Here's how the part is built. I have some questions about the finished solid (model axes, mm). A direction names the side the tool comes from. Coordinates: 2 decimals unless noted, no trailing zeros. Write each loop counter-clockwise with the first axis right and the second up, starting at its lowest first coordinate (ties: lowest second). Pieces come first, ordered by that corner, then holes. Notation, with made-up numbers: (22.25, 64) -> (57.25, 64) arc R11 ccw to (57.25, 71) -> close; hole circle Ø8 at (84.5, -25). An arc over 180 degrees is marked (long way). Use a Markdown table: item, result. Add a question column.
Item 1: If I drill on line 1 along X through (y, z) = (-23.5, -3.75); line 2 along Y through (x, z) = (0, -1.65); line 3 along X through (y, z) = (16, -1), over which ranges is the centre line in solid material (lowest first)? Write a range as from..to.
Item 2: Imagine slicing it at D-D, the plane y = 16. Write out the boundary of the cut face in (x, z).
Item 3: Will these pins go through, and if not, where does the flat tip stop? pin 1 Ø3 at (x, z) = (-37.5, -5) entering from -Y; pin 2 Ø4 at (x, z) = (36.5, -2) entering from +Y.
Item 4: On a 3-axis mill with a long thin cutter (end or side, diameter ignored), from which of +Z, -Z, +X, -X, +Y, -Y can I reach the whole of each face in a straight line? I mean faces 1 (the flat face through (13, -40, -4)), 2 (the cylindrical face through (-27.496, -24.628, -3.944)). Say none if no direction works.
Item 5: If we mould it in two halves opening along X, with no side actions, what happens to faces 3 (the cylindrical face through (20.21, -9.15, -3.94)), 4 (the flat face through (-1, -46, 0)), 5 (the cylindrical face through (-55.55, -42.594, -3.944))? For each: pulls with the +X half, pulls with the -X half, needs draft (parallel to the pull), parting line crosses it, or undercut.
Item 6: Imagine slicing it at A-A, the plane z = -2. Count the separate pieces of the cut face and the enclosed holes in it, and give its area (3 significant figures).
Item 7: Imagine slicing it at C-C, the plane x = 32. Write out the boundary of the cut face in (y, z), and give its area (3 significant figures).
Item 8: Imagine slicing it at B-B, the plane y = 0. Write out the boundary of the cut face in (x, z), and give its area (3 significant figures).
```python
from build123d import *

# Parameters (mm, degrees)
SKETCH_1_R          = 70
SKETCH_1_R_2        = 17.7
SKETCH_1_R_3        = 2.75
SKETCH_1_R_4        = 1.5
EXTRUDE_1_DEPTH     = 8
SKETCH_2_R          = 45.2
SKETCH_2_R_2        = 41.8
CUT_EXTRUDE_2_DEPTH = 4


with BuildPart() as part:
    # 草图1 → 凸台-拉伸1 (new body)
    with BuildSketch(Plane.XY):
        Circle(SKETCH_1_R)
        Circle(SKETCH_1_R_2, mode=Mode.SUBTRACT)
        with Locations((24.748737342, 24.748737342)):
            Circle(SKETCH_1_R_3, mode=Mode.SUBTRACT)
        with Locations((-24.748737342, 24.748737342)):
            Circle(SKETCH_1_R_3, mode=Mode.SUBTRACT)
        with Locations((-24.748737342, -24.748737342)):
            Circle(SKETCH_1_R_3, mode=Mode.SUBTRACT)
        with Locations((24.748737342, -24.748737342)):
            Circle(SKETCH_1_R_3, mode=Mode.SUBTRACT)
        with Locations((0, 23.75)):
            Circle(SKETCH_1_R_3, mode=Mode.SUBTRACT)
        with Locations((-20.56810334, -11.875)):
            Circle(SKETCH_1_R_3, mode=Mode.SUBTRACT)
        with Locations((20.56810334, -11.875)):
            Circle(SKETCH_1_R_3, mode=Mode.SUBTRACT)
        with Locations((0, 48)):
            Circle(SKETCH_1_R_4, mode=Mode.SUBTRACT)
    extrude(amount=-EXTRUDE_1_DEPTH)

    # 草图2 → 切除-拉伸2 (cut)
    with BuildSketch(Plane.XY):
        Circle(SKETCH_2_R)
        Circle(SKETCH_2_R_2, mode=Mode.SUBTRACT)
    extrude(amount=-CUT_EXTRUDE_2_DEPTH, mode=Mode.SUBTRACT)


solid = part.part
```
Ans:
| question | item | result |
|---|---|---|
| 1 | line 1 | x = -65.94..-38.61, -34.57..-27.2, -22.3..22.3, 27.2..34.57, 38.61..65.94 |
| 1 | line 2 | y = -70..-45.2, -41.8..-17.7, 17.7..21, 26.5..41.8, 45.2..46.5, 49.5..70 |
| 1 | line 3 | x = -68.15..-42.27, -38.62..-7.57, 7.57..38.62, 42.27..68.15 |
| 2 | outline | (-68.15, -8) -> (-7.57, -8) -> (-7.57, 0) -> (-38.62, 0) -> (-38.62, -4) -> (-42.27, -4) -> (-42.27, 0) -> (-68.15, 0) -> close; (7.57, -8) -> (68.15, -8) -> (68.15, 0) -> (42.27, 0) -> (42.27, -4) -> (38.62, -4) -> (38.62, 0) -> (7.57, 0) -> close |
| 3 | pin 1 | stops at y = -60.03 |
| 3 | pin 2 | stops at y = 60.91 |
| 4 | face 1 | +Z |
| 4 | face 2 | +Z, -Z |
| 5 | face 3 | undercut |
| 5 | face 4 | needs draft |
| 5 | face 5 | parting line crosses it |
| 6 | separate pieces | 2 |
| 6 | enclosed holes | 10 |
| 6 | area | 13,300 mm^2 |
| 7 | outline | (-62.26, -8) -> (62.26, -8) -> (62.26, 0) -> (31.92, 0) -> (31.92, -4) -> (26.89, -4) -> (26.89, 0) -> (-26.89, 0) -> (-26.89, -4) -> (-31.92, -4) -> (-31.92, 0) -> (-62.26, 0) -> close |
| 7 | area | 956 mm^2 |
| 8 | outline | (-70, -8) -> (-17.7, -8) -> (-17.7, 0) -> (-41.8, 0) -> (-41.8, -4) -> (-45.2, -4) -> (-45.2, 0) -> (-70, 0) -> close; (17.7, -8) -> (70, -8) -> (70, 0) -> (45.2, 0) -> (45.2, -4) -> (41.8, -4) -> (41.8, 0) -> (17.7, 0) -> close |
| 8 | area | 810 mm^2 |
